The figure shows three views and two pictorial views of one solid part (mm, origin at its lowest corner). Answer the questions. A direction names the side the tool comes from. Round coordinates to 2 decimals unless told otherwise and drop trailing zeros. Order: outer loops, then holes, each group sorted by start corner. A loop starts at its lowest first (then second) coordinate and runs counter-clockwise, first axis right, second up. Notation, with made-up numbers: (75.5, -39) - (104.5, -39) arc R22 cw to (104.5, -8) - close; hole circle Ø11 at (55, 84.5). An arc over 180 degrees is marked (long way). Use CSV: the item, a comma, the result in double quotes. Start each with the question number.
Item 1: Find section D-D, the plane x = 1.25. Give the vertices of the cut face in (y, z) (1 decimal).
Item 2: Straight lines are drawn through the part: line 1 along Y through (x, z) = (7, 6.35) (1 decimal); line 2 along Y through (x, z) = (7, 12) (1 decimal); line 3 along Y through (x, z) = (1, 8) (1 decimal). For each, find the intervals that lie inside material, in ascending order. Write a range as [from, to].
Item 3: Find section C-C, the plane y = 25.5. Give the vertices of the cut face in (x, z).
Item 4: Flat-ended cylindrical pins translate along their axes: P1, Ø4, axis at x = 7.5, z = 7, coming from the -Y side; P2, Ø6, axis at x = 10.5, y = 37, coming from the +Z side; P3, Ø5, axis at x = 4, y = 30.5, coming from the -Z side; P4, Ø6, axis at y = 6.35, z = 6.35, coming from the +X side (1 decimal). Find the tip coordinate at first contact, or state that the pin passes through.
Item 5: Find section A-A, the plane z = 6.35. Give the vertices of the cut face in (x, y) (1 decimal).
Item 6: For the marked faces 1, 2, 3 and 4, determine the directions among +Z, -Z, +X, -X, +Y, -Y from which every point of the face is accessible in a straight line to the end or side of a thin tool.
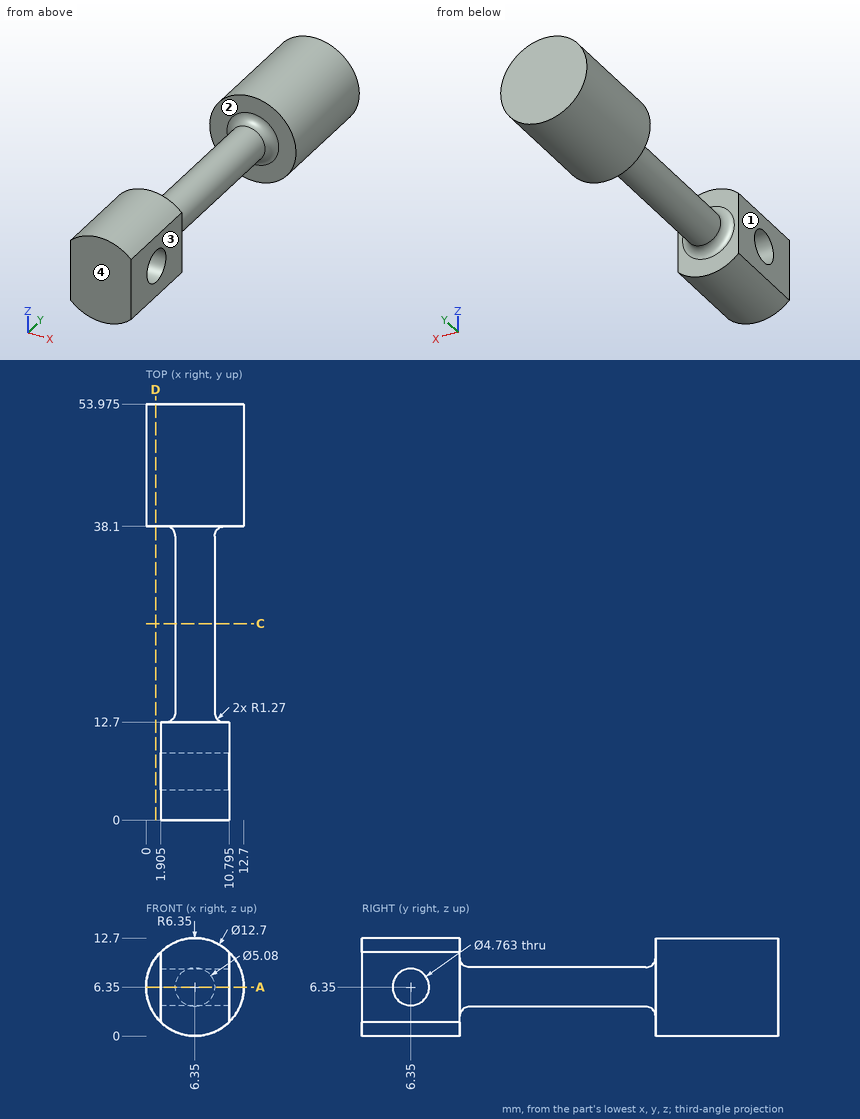
Worked out:
1,outline,"(38.1, 2.6) - (54, 2.6) - (54, 10.1) - (38.1, 10.1) - close"
2,line 1,"y = [0, 4], [8.7, 54]"
2,line 2,"y = [0, 12.7], [38.1, 54]"
2,line 3,"y = [38.1, 54]"
3,outline,"circle Ø5.08 at (6.35, 6.35)"
4,P1,"stops at y = 0"
4,P2,"stops at z = 12.55"
4,P3,"stops at z = 3.81"
4,P4,"stops at x = 10.8"
5,outline,"(0, 38.1) - (2.5, 38.1) arc R1.3 cw to (3.8, 36.8) - (3.8, 14) arc R1.3 cw to (2.5, 12.7) - (1.9, 12.7) - (1.9, 8.7) - (10.8, 8.7) - (10.8, 12.7) - (10.2, 12.7) arc R1.3 cw to (8.9, 14) - (8.9, 36.8) arc R1.3 cw to (10.2, 38.1) - (12.7, 38.1) - (12.7, 54) - (0, 54) - close; (1.9, 0) - (10.8, 0) - (10.8, 4) - (1.9, 4) - close"
6,face 1,"+Z, -Z, -X, -Y"
6,face 2,"none"
6,face 3,"+Z, -Z, +X, -Y"
6,face 4,"+Z, -Z, +X, -X, -Y"
